Could you check a few things on this model? Use its own coordinates, in mm. Give positions to 0.01 mm unless a question says otherwise; leave off trailing zeros. Write each loop counter-clockwise with the first axis right and the second up, starting at its lowest first coordinate (ties: lowest second). Pieces come first, ordered by that corner, then holes. Notation, with made-up numbers: (88, -20.75) - (140, -20.75) arc R27 ccw to (140, -0.75) - close; hole circle Ø1 at (-32, 22.5). An arc over 180 degrees is marked (long way). Use one line per item in the form item = value.
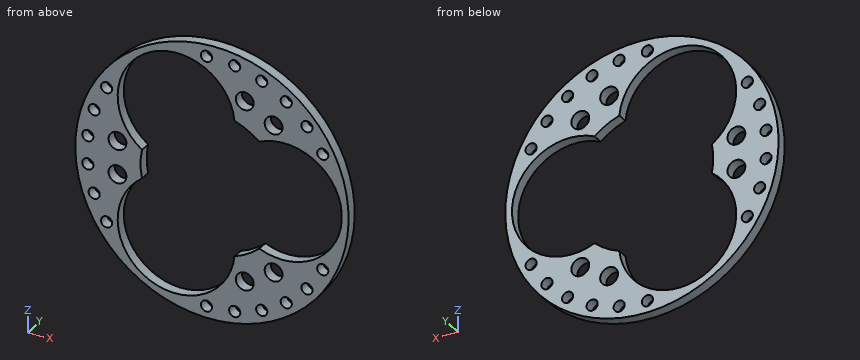
```python
from build123d import *

# Parameters (mm, degrees)
SKETCH1_R           = 122.5
SKETCH1_R_2         = 5
SKETCH1_R_3         = 8
BOSS_EXTRUDE1_DEPTH = 10


with BuildPart() as part:
    # Sketch1 → Boss-Extrude1 (new body)
    with BuildSketch(Plane(origin=(0, 0, 0), x_dir=(1, 0, 0), z_dir=(0, 1, 0))):
        with Locations(Location((0.129975876, -0.519903504, 0), (0, 0, 270))):
            Circle(SKETCH1_R)
        with Locations(Location((-105.445871126, 36.866464731, 0), (0, 0, 270))):
            Circle(SKETCH1_R_2, mode=Mode.SUBTRACT)
        with Locations(Location((-111.15007196, 12.158856438, 0), (0, 0, 270))):
            Circle(SKETCH1_R_2, mode=Mode.SUBTRACT)
        with Locations(Location((-84.563490883, 14.413839776, 0), (0, 0, 270))):
            Circle(SKETCH1_R_3, mode=Mode.SUBTRACT)
        with Locations(Location((-84.563490883, -15.453646783, 0), (0, 0, 270))):
            Circle(SKETCH1_R_3, mode=Mode.SUBTRACT)
        with Locations(Location((-105.445871126, -37.906271738, 0), (0, 0, 270))):
            Circle(SKETCH1_R_2, mode=Mode.SUBTRACT)
        with Locations(Location((-111.15007196, -13.198663446, 0), (0, 0, 270))):
            Circle(SKETCH1_R_2, mode=Mode.SUBTRACT)
        with Locations(Location((-94.329866055, 59.657652631, 0), (0, 0, 270))):
            Circle(SKETCH1_R_2, mode=Mode.SUBTRACT)
        with Locations(Location((-4.755395509, 111.373497314, 0), (0, 0, 270))):
            Circle(SKETCH1_R_2, mode=Mode.SUBTRACT)
        with Locations(Location((20.540354731, 109.604646144, 0), (0, 0, 270))):
            Circle(SKETCH1_R_2, mode=Mode.SUBTRACT)
        with Locations(Location((-4.755395509, -112.413304321, 0), (0, 0, 270))):
            Circle(SKETCH1_R_2, mode=Mode.SUBTRACT)
        with Locations(Location((20.540354731, -110.644453151, 0), (0, 0, 270))):
            Circle(SKETCH1_R_2, mode=Mode.SUBTRACT)
        with Locations(Location((44.789871596, -103.230631835, 0), (0, 0, 270))):
            Circle(SKETCH1_R_2, mode=Mode.SUBTRACT)
        with Locations(Location((66.750127992, -90.551871893, 0), (0, 0, 270))):
            Circle(SKETCH1_R_2, mode=Mode.SUBTRACT)
        with Locations(Location((85.295444023, -73.258084917, 0), (0, 0, 270))):
            Circle(SKETCH1_R_2, mode=Mode.SUBTRACT)
        with Locations(Location((99.475189192, -52.235748186, 0), (0, 0, 270))):
            Circle(SKETCH1_R_2, mode=Mode.SUBTRACT)
        with Locations(Location((55.409710309, -66.399725612, 0), (0, 0, 270))):
            Circle(SKETCH1_R_3, mode=Mode.SUBTRACT)
        with Locations(Location((29.543708202, -81.333468891, 0), (0, 0, 270))):
            Circle(SKETCH1_R_3, mode=Mode.SUBTRACT)
        with Locations(Location((-94.329866055, -60.697459638, 0), (0, 0, 270))):
            Circle(SKETCH1_R_2, mode=Mode.SUBTRACT)
        with Locations(Location((29.543708202, 80.293661884, 0), (0, 0, 270))):
            Circle(SKETCH1_R_3, mode=Mode.SUBTRACT)
        with Locations(Location((55.409710309, 65.359918605, 0), (0, 0, 270))):
            Circle(SKETCH1_R_3, mode=Mode.SUBTRACT)
        with Locations(Location((99.475189192, 51.195941179, 0), (0, 0, 270))):
            Circle(SKETCH1_R_2, mode=Mode.SUBTRACT)
        with Locations(Location((85.295444023, 72.218277909, 0), (0, 0, 270))):
            Circle(SKETCH1_R_2, mode=Mode.SUBTRACT)
        with Locations(Location((66.750127992, 89.512064886, 0), (0, 0, 270))):
            Circle(SKETCH1_R_2, mode=Mode.SUBTRACT)
        with Locations(Location((44.789871596, 102.190824828, 0), (0, 0, 270))):
            Circle(SKETCH1_R_2, mode=Mode.SUBTRACT)
        with BuildLine():
            ThreePointArc((20.36256799, 60.197822214), (-58.120024124, 100.372056037), (-62.569413113, 12.317020601))
            ThreePointArc((-62.569413113, 12.317020601), (-63.870024124, -0.519903504), (-62.569413113, -13.356827608))
            ThreePointArc((-62.569413113, -13.356827608), (-58.120024124, -101.411863045), (20.36256799, -61.237629222))
            ThreePointArc((20.36256799, -61.237629222), (32.129975876, -55.945529346), (42.596772751, -48.400705117))
            ThreePointArc((42.596772751, -48.400705117), (116.629975876, -0.519903504), (42.596772751, 47.36089811))
            ThreePointArc((42.596772751, 47.36089811), (32.129975876, 54.905722339), (20.36256799, 60.197822214))
        make_face(mode=Mode.SUBTRACT)
    extrude(amount=BOSS_EXTRUDE1_DEPTH)


solid = part.part
```
1. Imagine slicing it at B-B, the plane y = 7. State how many separate pieces and enclosed holes the cut face has, and give its area (3 significant figures).
Response values:
separate_pieces = 1
enclosed_holes = 25
area = 16,400 mm²
2. Imagine slicing it at A-A, the plane z = 29. List the corners of the cut face in (x, y) for me.
Response values:
outline = (-119.01, 0) - (-76.93, 0) - (-76.93, 10) - (-119.01, 10) - close; (108.23, 0) - (119.27, 0) - (119.27, 10) - (108.23, 10) - close
3. If I drill on line 1 (X direction, y = 5.5, z = -81.5); line 2 (X direction, y = 6.5, z = 62); line 3 (X direction, y = 3.75, z = 79.5), over which ranges is the centre line in solid material (lowest first)? Write a range as from..to.
Response values:
line_1 = -90.86..-77.14, 13.4..21.64, 37.45..91.12
line_2 = -105.82..-99.16, -89.5..-84.02, 20.28..48.73, 62.09..106.08
line_3 = -93.51..-78.79, 15.05..21.76, 37.33..93.77
4. For pin 1 (1.5 mm diameter, centred on y = 4, z = -74.5, fed in from -X); pin 2 (13 mm diameter, centred on x = 29.54, z = 81.33, fed in from +Y); pin 3 (18.5 mm diameter, centred on x = -84.56, z = -14.41, fed in from +Y); pin 4 (1.5 mm diameter, centred on x = -22.5, y = 2, fed in from -Z), each with a flat end and sliding along its axis, tell me the tip position at first contact or that it passes through.
Response values:
pin_1 = -97.29
pin_2 = through
pin_3 = 10
pin_4 = -120.01
